The listing builds one solid part. Answer for the finished solid, in the listing's coordinates (mm). A direction names the side the tool comes from. Give positions to 0.01 mm unless a question says otherwise; leave off trailing zeros. Order: outer loops, then holes, each group sorted by start corner. A loop starts at its lowest first (then second) coordinate and runs counter-clockwise, first axis right, second up. Notation, with made-up numbers: (47, -34.75) -> (58, -34.75) arc R20 ccw to (58, -5.75) -> close; hole circle Ø3 at (57.25, 86.5). An arc over 180 degrees is marked (long way). Write item = value, one per line. Start each with the question number.
```python
from build123d import *

# Parameters (mm, degrees)
SKETCH_1_W          = 15
SKETCH_1_H          = 19
SKETCH_1_R          = 1.1
EXTRUDE_1_DEPTH     = 4
SKETCH_2_R          = 1.8
CUT_EXTRUDE_1_DEPTH = 2
FILLET_1_R          = 1


with BuildPart() as part:
    # Эскиз1 → Бобышка-Вытянуть1 (new body)
    with BuildSketch(Plane(origin=(0, 0, 0), x_dir=(0, 0, -1), z_dir=(1, 0, 0))):
        Rectangle(SKETCH_1_W, SKETCH_1_H)
        with Locations((0, 5)):
            Circle(SKETCH_1_R, mode=Mode.SUBTRACT)
        with Locations((0, -5)):
            Circle(SKETCH_1_R, mode=Mode.SUBTRACT)
    extrude(amount=EXTRUDE_1_DEPTH)

    # Эскиз2 → Вырез-Вытянуть1 (cut)
    with BuildSketch(Plane(origin=(4, 0, 0), x_dir=(0, 0, -1), z_dir=(1, 0, 0))):
        with Locations((0, 5)):
            Circle(SKETCH_2_R)
        with Locations((0, -5)):
            Circle(SKETCH_2_R)
    extrude(amount=-CUT_EXTRUDE_1_DEPTH, mode=Mode.SUBTRACT)

    # Скругление1
    fillet_1_edges = [part.edges().sort_by_distance(p)[0] for p in [
        (4, -9.5, 0),
        (4, 9.5, 0),
    ]]
    fillet(fillet_1_edges, radius=FILLET_1_R)


solid = part.part
```
Item 1: Consider L1, parallel to Y at x = 2.65, z = 0; L2, parallel to Y at x = 0.9, z = 0; L3, parallel to Z at x = 0.55, y = 5. Determine where each line is inside the solid, lowest interval first. Write a range as from..to.
Item 2: A cutting plane is placed at C-C, the plane x = 1. Write down the section's boundary in (y, z).
Item 3: A cutting plane is placed at D-D, the plane z = -1.5. Write down the section's boundary in (x, y).
Item 4: The mould has two halves that part along Z. Classify faces 3 (the flat face through (4, 0, 0)), 4 (the flat face through (2, 0, 7.5)), 5 (the cylindrical face through (0.99, -4.07, -0.59)): +Z half, -Z half, draft (parallel to the pull), parting line (faces both ways), or undercut.
Item 5: A flat-ended cylindrical pin translates along its axis: pin 1 (3 mm diameter, centred on y = -5, z = 0, fed in from +X). Find the tip coordinate at first contact, or state that the pin passes through.
Item 6: A cutting plane is placed at B-B, the plane z = 0. Write down the section's boundary in (x, y).
Item 7: Which of the six approach directions +Z, -Z, +X, -X, +Y, -Y give full straight-line access (tool end or side, diameter ignored) to faces 1 (the flat face through (1, 9.5, 0)), 2 (the flat face through (2, 6, -1))?
Item 8: A cutting plane is placed at A-A, the plane y = -5. Write down the section's boundary in (x, z), plus the area to 3 significant figures.
Check values:
q1.L1 = -9.5..-6.8, -3.2..3.2, 6.8..9.5
q1.L2 = -9.5..-6.1, -3.9..3.9, 6.1..9.5
q1.L3 = -7.5..-1.1, 1.1..7.5
q2.outline = (-9.5, -7.5) -> (9.5, -7.5) -> (9.5, 7.5) -> (-9.5, 7.5) -> close; hole circle Ø2.2 at (-5, 0); hole circle Ø2.2 at (5, 0)
q3.outline = (0, -9.5) -> (3, -9.5) arc R1 ccw to (4, -8.5) -> (4, -5.99) -> (2, -5.99) -> (2, -4.01) -> (4, -4.01) -> (4, 4.01) -> (2, 4.01) -> (2, 5.99) -> (4, 5.99) -> (4, 8.5) arc R1 ccw to (3, 9.5) -> (0, 9.5) -> close
q4.face_3 = draft
q4.face_4 = +Z half
q4.face_5 = undercut
q5.pin_1 = 2
q6.outline = (0, -9.5) -> (3, -9.5) arc R1 ccw to (4, -8.5) -> (4, -6.8) -> (2, -6.8) -> (2, -6.1) -> (0, -6.1) -> close; (0, -3.9) -> (2, -3.9) -> (2, -3.2) -> (4, -3.2) -> (4, 3.2) -> (2, 3.2) -> (2, 3.9) -> (0, 3.9) -> close; (0, 6.1) -> (2, 6.1) -> (2, 6.8) -> (4, 6.8) -> (4, 8.5) arc R1 ccw to (3, 9.5) -> (0, 9.5) -> close
q7.face_1 = +Z, -Z, +X, -X, +Y
q7.face_2 = +X
q8.outline = (0, -7.5) -> (4, -7.5) -> (4, -1.8) -> (2, -1.8) -> (2, -1.1) -> (0, -1.1) -> close; (0, 1.1) -> (2, 1.1) -> (2, 1.8) -> (4, 1.8) -> (4, 7.5) -> (0, 7.5) -> close
q8.area = 48.4 mm^2
